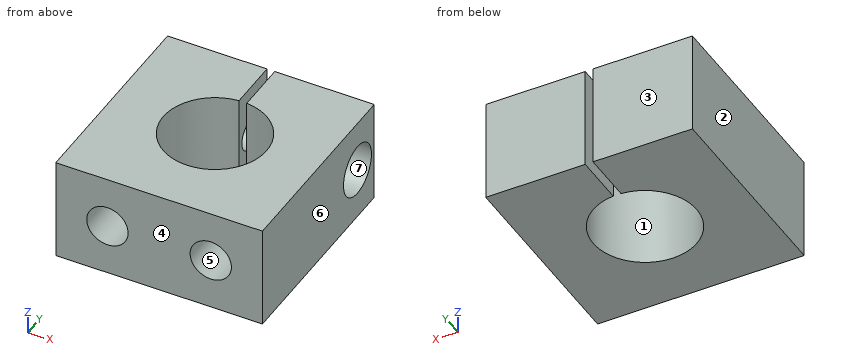
from build123d import *

# Parameters (mm, degrees)
CROQUIS1_R              = 3
SALIENTE_EXTRUIR1_DEPTH = 20
CROQUIS2_R              = 3
CORTAR_EXTRUIR1_DEPTH   = 30
CROQUIS3_R              = 5
CORTAR_EXTRUIR2_DEPTH   = 10
CROQUIS4_W              = 40
CROQUIS4_H              = 50
CORTAR_EXTRUIR3_DEPTH   = 54.150729064
CROQUIS5_R              = 4
CORTAR_EXTRUIR4_DEPTH   = 10


with BuildPart() as part:
    # Croquis1 → Saliente-Extruir1 (new body)
    with BuildSketch(Plane.XY):
        with BuildLine():
            Line((-0.75, 34.971835338), (-0.75, 45))
            Line((-0.75, 45), (-20, 45))
            Line((-20, 45), (-20, -45))
            Line((-20, -45), (20, -45))
            Line((20, -45), (20, 45))
            Line((20, 45), (0.75, 45))
            Line((0.75, 45), (0.75, 34.971835338))
            ThreePointArc((0.75, 34.971835338), (0, 15), (-0.75, 34.971835338))
        make_face()
        with Locations((-10, -35)):
            Circle(CROQUIS1_R, mode=Mode.SUBTRACT)
        with Locations((10, -35)):
            Circle(CROQUIS1_R, mode=Mode.SUBTRACT)
    extrude(amount=SALIENTE_EXTRUIR1_DEPTH)

    # Croquis2 → Cortar-Extruir1 (cut)
    with BuildSketch(Plane(origin=(20, 0, 0), x_dir=(0, 0, -1), z_dir=(1, 0, 0))):
        with Locations((-10, 39)):
            Circle(CROQUIS2_R)
    extrude(amount=-CORTAR_EXTRUIR1_DEPTH, mode=Mode.SUBTRACT)

    # Croquis3 → Cortar-Extruir2 (cut)
    with BuildSketch(Plane(origin=(20, 0, 0), x_dir=(0, 0, -1), z_dir=(1, 0, 0))):
        with Locations((-10, 39)):
            Circle(CROQUIS3_R)
    extrude(amount=-CORTAR_EXTRUIR2_DEPTH, mode=Mode.SUBTRACT)

    # Croquis4 → Cortar-Extruir3 (cut, through all)
    with BuildSketch(Plane.XY.offset(20)):
        with Locations((0, -20)):
            Rectangle(CROQUIS4_W, CROQUIS4_H)
    extrude(amount=-CORTAR_EXTRUIR3_DEPTH, mode=Mode.SUBTRACT)

    # Croquis5 → Cortar-Extruir4 (cut)
    with BuildSketch(Plane.XZ.offset(-5)):
        with Locations(Location((-10, 10, 0), (0, 0, 270))):
            Circle(CROQUIS5_R)
        with Locations(Location((10, 10, 0), (0, 0, 270))):
            Circle(CROQUIS5_R)
    extrude(amount=-CORTAR_EXTRUIR4_DEPTH, mode=Mode.SUBTRACT)


solid = part.part
Geometry: final body of the model. Coordinates: model frame, mm. Face numbers are marked on the shaded views. A direction names the side the tool comes from. Round coordinates to 2 decimals unless told otherwise and drop trailing zeros. Order: outer loops, then holes, each group sorted by start corner. A loop starts at its lowest first (then second) coordinate and runs counter-clockwise, first axis right, second up. Notation, with made-up numbers: (-2, 23) -> (3, 23) arc R14 ccw to (3, 38) -> close; hole circle Ø4 at (-2, 36). An arc over 180 degrees is marked (long way). Put each result on its own line as item: value. Start each with the question number.
Q1. Section C-C on y = 39. Return the cut outline in (x, z).
Q2. Reachability of the marked faces 5, 6 and 7 from +Z, -Z, +X, -X, +Y, -Y: full face, straight path, thin tool, end or side. Return the list, or none.
Q3. Pull-direction query (Y, two-part tool) for the marked faces 1, 2, 3 and 4; classes: +Y half, -Y half, draft (parallel to the pull), parting line (faces both ways), or undercut.
Q4. First-contact query: pin 1 (3.5 mm diameter, centred on y = 39, z = 10, fed in from +X). Flat tip, straight axial feed; report the tip coordinate or a pass-through.
Q5. Section D-D on x = 9. Return the cut outline in (y, z).
Q6. Line query: probe 1 along X at (y, z) = (8.75, 10); probe 2 along Y at (x, z) = (12, 10); probe 3 along Y at (x, z) = (16, 10). Output: solid intervals per line, ascending.
Q7. Section A-A on y = 17. Return the cut outline in (x, z), and give its area (3 significant figures).
Q8. Section B-B on z = 10. Return the cut outline in (x, y).
Ans:
1. outline: (-20, 0) -> (-0.75, 0) -> (-0.75, 7) -> (-10, 7) -> (-10, 13) -> (-0.75, 13) -> (-0.75, 20) -> (-20, 20) -> close; (0.75, 0) -> (20, 0) -> (20, 5) -> (10, 5) -> (10, 7) -> (0.75, 7) -> close; (0.75, 13) -> (10, 13) -> (10, 15) -> (20, 15) -> (20, 20) -> (0.75, 20) -> close
2. face 5: -Y
2. face 6: +Z, -Z, +X, +Y, -Y
2. face 7: +X
3. face 1: undercut
3. face 2: draft
3. face 3: +Y half
3. face 4: -Y half
4. pin 1: stops at x = -10
5. outline: (5, 0) -> (20.64, 0) -> (20.64, 20) -> (5, 20) -> (5, 13.87) -> (15, 13.87) -> (15, 6.13) -> (5, 6.13) -> close; (29.36, 0) -> (45, 0) -> (45, 20) -> (29.36, 20) -> close; hole circle Ø6 at (39, 10)
6. probe 1: x = -20 to -14, -6 to 6, 14 to 20
6. probe 2: y = 15 to 34, 44 to 45
6. probe 3: y = 5 to 34, 44 to 45
7. outline: (-20, 0) -> (-6, 0) -> (-6, 20) -> (-20, 20) -> close; (6, 0) -> (20, 0) -> (20, 20) -> (6, 20) -> close
7. area: 560 mm2
8. outline: (-20, 5) -> (-14, 5) -> (-14, 15) -> (-6, 15) -> (-6, 5) -> (6, 5) -> (6, 15) -> (14, 15) -> (14, 5) -> (20, 5) -> (20, 34) -> (10, 34) -> (10, 36) -> (0.75, 36) -> (0.75, 34.97) arc R10 cw (long way) to (-0.75, 34.97) -> (-0.75, 36) -> (-10, 36) -> (-10, 42) -> (-0.75, 42) -> (-0.75, 45) -> (-20, 45) -> close; (0.75, 42) -> (10, 42) -> (10, 44) -> (20, 44) -> (20, 45) -> (0.75, 45) -> close
